from build123d import *

# Parameters (mm, degrees)
SKETCH_1_R          = 1.6
EXTRUDE_4_DEPTH     = 13
EXTRUDE_4_2_DEPTH   = 13
EXTRUDE_4_3_DEPTH   = 13
EXTRUDE_4_4_DEPTH   = 13
SKETCH_1_R_2        = 2.1
EXTRUDE_4_5_DEPTH   = 13
EXTRUDE_4_6_DEPTH   = 13
EXTRUDE_4_7_DEPTH   = 13
SKETCH_8_R          = 49
EXTRUDE_5_DEPTH     = 3
SKETCH_9_R          = 2.1
CUT_EXTRUDE_2_DEPTH = 13
SKETCH_3_R          = 8.6
CUT_EXTRUDE_3_DEPTH = 13
SKETCH_6_R          = 4.05
CUT_EXTRUDE_4_DEPTH = 13
CUT_EXTRUDE_5_DEPTH = 13
SKETCH_2_R          = 11.5
CUT_EXTRUDE_6_DEPTH = 13
FILLET_1_R          = 2
CUT_EXTRUDE_7_REACH = 71.361
SKETCH_10_R         = 2.25
EXTRUDE_START       = -3
SKETCH_11_R         = 2.1
EXTRUDE_6_DEPTH     = 3


with BuildPart() as part:
    # Sketch 1 → Extrude 4 (new body)
    with BuildSketch(Plane.XY):
        with Locations((0, 44)):
            Circle(SKETCH_1_R)
    extrude(amount=EXTRUDE_4_DEPTH)



with BuildPart() as body_2:
    # Sketch 1 → Extrude 4 2 (new body)
    with BuildSketch(Plane.XY):
        with Locations((44, 0)):
            Circle(SKETCH_1_R)
    extrude(amount=EXTRUDE_4_2_DEPTH)


with BuildPart() as body_3:
    # Sketch 1 → Extrude 4 3 (new body)
    with BuildSketch(Plane.XY):
        with Locations((0, -44)):
            Circle(SKETCH_1_R)
    extrude(amount=EXTRUDE_4_3_DEPTH)


with BuildPart() as body_4:
    # Sketch 1 → Extrude 4 4 (new body)
    with BuildSketch(Plane.XY):
        with Locations((-44, 0)):
            Circle(SKETCH_1_R)
    extrude(amount=EXTRUDE_4_4_DEPTH)


with BuildPart() as body_5:
    # Sketch 1 → Extrude 4 5 (new body)
    with BuildSketch(Plane.XY):
        with Locations((29, 0)):
            Circle(SKETCH_1_R_2)
    extrude(amount=EXTRUDE_4_5_DEPTH)


with BuildPart() as body_6:
    # Sketch 1 → Extrude 4 6 (new body)
    with BuildSketch(Plane.XY):
        with Locations((-14.5, 25.11473671)):
            Circle(SKETCH_1_R_2)
    extrude(amount=EXTRUDE_4_6_DEPTH)


with BuildPart() as body_7:
    # Sketch 1 → Extrude 4 7 (new body)
    with BuildSketch(Plane.XY):
        with Locations((-14.5, -25.11473671)):
            Circle(SKETCH_1_R_2)
    extrude(amount=EXTRUDE_4_7_DEPTH)


with BuildPart() as part_1:
    add(part.part)

    add(body_2.part)  # Extrude 5 merges body 2

    add(body_3.part)  # Extrude 5 merges body 3

    add(body_4.part)  # Extrude 5 merges body 4

    add(body_5.part)  # Extrude 5 merges body 5

    add(body_6.part)  # Extrude 5 merges body 6

    add(body_7.part)  # Extrude 5 merges body 7
    # Sketch 8 → Extrude 5 (add)
    with BuildSketch(Plane.XY):
        Circle(SKETCH_8_R)
    extrude(amount=EXTRUDE_5_DEPTH)

    # Sketch 9 → Cut-Extrude 2 (cut)
    with BuildSketch(Plane.XY):
        with Locations((0, 44)):
            Circle(SKETCH_9_R)
        with Locations((44, 0)):
            Circle(SKETCH_9_R)
        with Locations((0, -44)):
            Circle(SKETCH_9_R)
        with Locations((-44, 0)):
            Circle(SKETCH_9_R)
        with Locations((-14.5, 25.11473671)):
            Circle(SKETCH_9_R)
        with Locations((-14.5, -25.11473671)):
            Circle(SKETCH_9_R)
        with Locations((29, 0)):
            Circle(SKETCH_9_R)
    extrude(amount=CUT_EXTRUDE_2_DEPTH, mode=Mode.SUBTRACT)

    # Sketch 3 → Cut-Extrude 3 (cut)
    with BuildSketch(Plane.XY):
        Circle(SKETCH_3_R)
    extrude(amount=CUT_EXTRUDE_3_DEPTH, mode=Mode.SUBTRACT)

    # Sketch 6 → Cut-Extrude 4 (cut)
    with BuildSketch(Plane.XY):
        with Locations((19.25, 0)):
            Circle(SKETCH_6_R)
    extrude(amount=CUT_EXTRUDE_4_DEPTH, mode=Mode.SUBTRACT)

    # Sketch 7 → Cut-Extrude 5 (cut)
    with BuildSketch(Plane.XY):
        Polygon((10.802199699, 10.505830841), (14.272482459, 16.5145615), (7.171657827, 20.615572296), (3.701375067, 14.606841637), align=None)
    extrude(amount=CUT_EXTRUDE_5_DEPTH, mode=Mode.SUBTRACT)

    # Sketch 2 → Cut-Extrude 6 (cut)
    with BuildSketch(Plane.XY):
        Circle(SKETCH_2_R)
    extrude(amount=CUT_EXTRUDE_6_DEPTH, mode=Mode.SUBTRACT)

    # Fillet 1
    fillet_1_edges = [part_1.edges().sort_by_distance(p)[0] for p in [
        (7.171657827, 20.615572296, 1.5),
        (3.701375067, 14.606841637, 1.5),
        (10.802199699, 10.505830841, 1.5),
        (14.272482459, 16.5145615, 1.5),
    ]]
    fillet(fillet_1_edges, radius=FILLET_1_R)

    # Sketch 10 → Cut-Extrude 7 (cut, up to next)
    with BuildSketch(Plane.XY.offset(3), mode=Mode.PRIVATE) as cut_extrude_7_sk1:
        with Locations((-31.112698372, 31.112698372)):
            Circle(SKETCH_10_R)
    cut_extrude_7_tool1 = extrude(cut_extrude_7_sk1.sketch, amount=-CUT_EXTRUDE_7_REACH, mode=Mode.PRIVATE) & part_1.part
    # Sketch 10 → Cut-Extrude 7 (cut, up to next)
    with BuildSketch(Plane.XY.offset(3), mode=Mode.PRIVATE) as cut_extrude_7_sk2:
        with Locations((31.112698372, 31.112698372)):
            Circle(SKETCH_10_R)
    cut_extrude_7_tool2 = extrude(cut_extrude_7_sk2.sketch, amount=-CUT_EXTRUDE_7_REACH, mode=Mode.PRIVATE) & part_1.part
    # Sketch 10 → Cut-Extrude 7 (cut, up to next)
    with BuildSketch(Plane.XY.offset(3), mode=Mode.PRIVATE) as cut_extrude_7_sk3:
        with Locations((31.112698372, -31.112698372)):
            Circle(SKETCH_10_R)
    cut_extrude_7_tool3 = extrude(cut_extrude_7_sk3.sketch, amount=-CUT_EXTRUDE_7_REACH, mode=Mode.PRIVATE) & part_1.part
    # Sketch 10 → Cut-Extrude 7 (cut, up to next)
    with BuildSketch(Plane.XY.offset(3), mode=Mode.PRIVATE) as cut_extrude_7_sk4:
        with Locations((-31.112698372, -31.112698372)):
            Circle(SKETCH_10_R)
    cut_extrude_7_tool4 = extrude(cut_extrude_7_sk4.sketch, amount=-CUT_EXTRUDE_7_REACH, mode=Mode.PRIVATE) & part_1.part
    add(cut_extrude_7_tool1.solids().sort_by_distance((-31.112698, 31.112698, 3))[0], mode=Mode.SUBTRACT)
    add(cut_extrude_7_tool2.solids().sort_by_distance((31.112698, 31.112698, 3))[0], mode=Mode.SUBTRACT)
    add(cut_extrude_7_tool3.solids().sort_by_distance((31.112698, -31.112698, 3))[0], mode=Mode.SUBTRACT)
    add(cut_extrude_7_tool4.solids().sort_by_distance((-31.112698, -31.112698, 3))[0], mode=Mode.SUBTRACT)

    # Sketch 11 → Extrude 6 (add)
    with BuildSketch(Plane.XY.offset(3).offset(EXTRUDE_START)):
        with Locations((-44, 0)):
            Circle(SKETCH_11_R)
        with Locations((0, -44)):
            Circle(SKETCH_11_R)
        with Locations((44, 0)):
            Circle(SKETCH_11_R)
        with Locations((0, 44)):
            Circle(SKETCH_11_R)
    extrude(amount=EXTRUDE_6_DEPTH)


solid = part_1.part
Geometry check sheet. Reference: the model listing, model coordinates, mm. A direction names the side the tool comes from. Give positions to 0.01 mm unless a question says otherwise; leave off trailing zeros. Order: outer loops, then holes, each group sorted by start corner. A loop starts at its lowest first (then second) coordinate and runs counter-clockwise, first axis right, second up. Notation, with made-up numbers: (47, 87) - (90, 87) arc R14 cw to (90, 99) - close; hole circle Ø8 at (-18, 26). An arc over 180 degrees is marked (long way). Answer as a JSON object with one key per item and string values.
(1) Material ranges on line 1 (Y direction, x = -30.5, z = 1.2); line 2 (X direction, y = -3.5, z = 2.5); line 3 (Y direction, x = -14.5, z = 1.55), recorded low to high.
Report:
{"line 1": "-38.35 to -33.28, -28.95 to 28.95, 33.28 to 38.35", "line 2": "-48.87 to -10.95, 10.95 to 17.21, 21.29 to 48.87", "line 3": "-46.81 to -27.21, -23.01 to 23.01, 27.21 to 46.81"}
(2) Cross-section at C-C (z = 0.7). State how many separate pieces and enclosed holes the cut face has, then the cut area to 3 significant figures.
Report:
{"separate pieces": "1", "enclosed holes": "10", "area": "6,920 mm^2"}
(3) Cross-section at D-D (x = -14.5). Record the cut outline in (y, z).
Report:
{"outline": "(-46.81, 0) - (-27.21, 0) - (-27.21, 3) - (-46.81, 3) - close; (-23.01, 0) - (23.01, 0) - (23.01, 3) - (-23.01, 3) - close; (27.21, 0) - (46.81, 0) - (46.81, 3) - (27.21, 3) - close"}
(4) Draft check along X on faces 3 (the cylindrical face through (26.34, 41.32, 1.48)), 4 (the cylindrical face through (7.41, 19.82, 1.52)), 5 (the flat face through (-12, 1, 3)). Enter one of: released by +X, released by -X, zero draft, split by the parting line, or undercut.
Report:
{"face 3": "split by the parting line", "face 4": "undercut", "face 5": "zero draft"}
(5) Cross-section at B-B (y = 0). Record the cut outline in (x, z).
Report:
{"outline": "(-49, 0) - (-11.5, 0) - (-11.5, 3) - (-49, 3) - close; (11.5, 0) - (15.2, 0) - (15.2, 3) - (11.5, 3) - close; (23.3, 0) - (26.9, 0) - (26.9, 3) - (23.3, 3) - close; (31.1, 0) - (49, 0) - (49, 3) - (31.1, 3) - close"}
(6) Depth check by flat-ended pin: pin 1 Ø7 at (x, y) = (31.11, -31.11) entering from +Z. Enter the tip coordinate at first touch or a pass-through.
Report:
{"pin 1": "z = 3"}
(7) Tool access check on faces 1 (the flat face through (12.527, 13.492, 1.479)), 2 (the flat face through (-12, 1, 0)). Record the directions out of +Z, -Z, +X, -X, +Y, -Y that give a thin tool (end or side, any length) a straight path to the whole face; none if there is none.
Report:
{"face 1": "+Z, -Z", "face 2": "-Z, +X, -X, +Y, -Y"}
(8) Cross-section at A-A (x = 0.5). Record the cut outline in (y, z).
Report:
{"outline": "(-49, 0) - (-11.49, 0) - (-11.49, 3) - (-49, 3) - close; (11.49, 0) - (49, 0) - (49, 3) - (11.49, 3) - close"}
